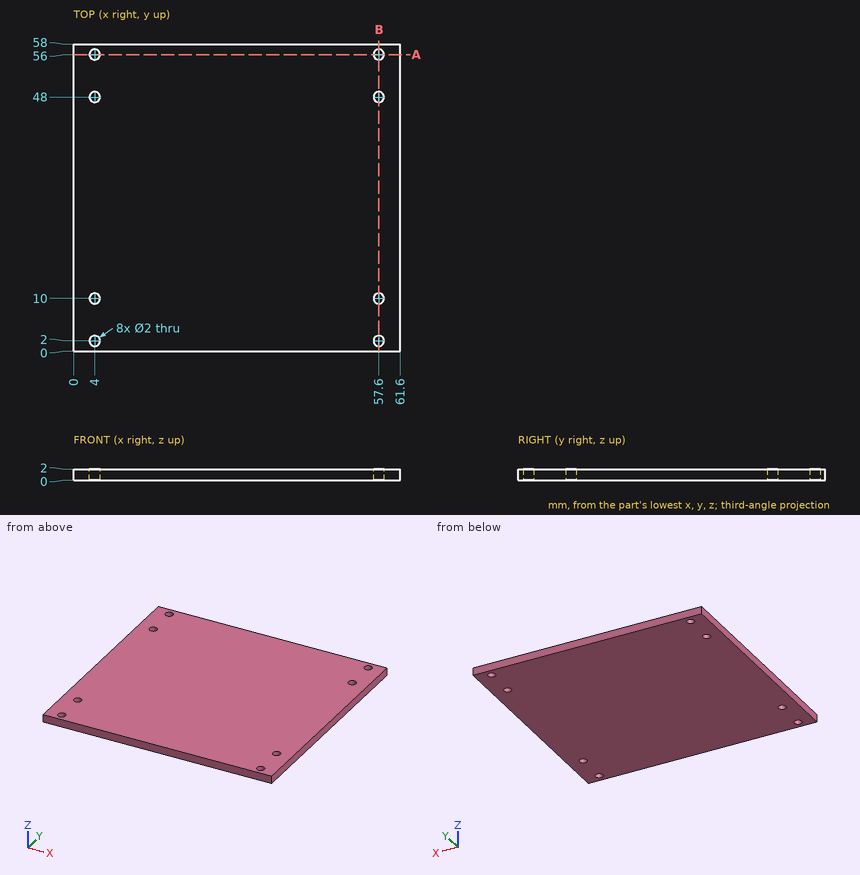
For this review, use the dimensioned drawing (mm, ordinates from the lowest corner) and the shaded views. Round coordinates to 2 decimals unless told otherwise and drop trailing zeros. Write each loop counter-clockwise with the first axis right and the second up, starting at its lowest first coordinate (ties: lowest second). Pieces come first, ordered by that corner, then holes. Notation, with made-up numbers: M 75,-17 L 123,-17 A21 cw 123,11 Z; hole C 82.25,38 d5. An arc over 180 degrees is marked long. Write item = value, one per line. Start each with the question number.
(1) For line 1 along Y through (x, z) = (4, 0.6); line 2 along X through (y, z) = (56, 0.7), list the stretches that pass through material, from the lowest coordinate up.
(2) We need section B-B (x = 57.6). Give the boundary of the cut face in (y, z), then the cut area to 3 significant figures.
(3) We need section A-A (y = 56). Give the boundary of the cut face in (x, z), then the cut area to 3 significant figures.
(4) Clearance check with flat-ended pins moving along their axes: pin 1 Ø1 at (x, z) = (49.5, 1.5) entering from -Y; pin 2 Ø1.8 at (x, y) = (57.6, 56) entering from +Z. State where each tip first meets the part, or that it passes through.
Results found:
q1.line_1 = 0 to 1, 3 to 9, 11 to 47, 49 to 55, 57 to 58
q1.line_2 = 0 to 3, 5 to 56.6, 58.6 to 61.6
q2.outline = M 0,0 L 1,0 L 1,2 L 0,2 Z; M 3,0 L 9,0 L 9,2 L 3,2 Z; M 11,0 L 47,0 L 47,2 L 11,2 Z; M 49,0 L 55,0 L 55,2 L 49,2 Z; M 57,0 L 58,0 L 58,2 L 57,2 Z
q2.area = 100 mm²
q3.outline = M 0,0 L 3,0 L 3,2 L 0,2 Z; M 5,0 L 56.6,0 L 56.6,2 L 5,2 Z; M 58.6,0 L 61.6,0 L 61.6,2 L 58.6,2 Z
q3.area = 115 mm²
q4.pin_1 = 0
q4.pin_2 = through
